For this review, take the finished solid that the model builds, in its own axes (mm). A direction names the side the tool comes from. Round coordinates to 2 decimals unless told otherwise and drop trailing zeros. Write each loop counter-clockwise with the first axis right and the second up, starting at its lowest first coordinate (ties: lowest second). Pieces come first, ordered by that corner, then holes. Notation, with made-up numbers: (43, 20.25) -> (51, 20.25) arc R22 cw to (51, 58.25) -> close; hole circle Ø7 at (33.25, 29). An arc over 180 degrees is marked (long way). Answer in a Markdown table with one row per item.
from build123d import *

# Parameters (mm, degrees)
SKETCH2_W               = 127
SKETCH2_H               = 63.5
BOSS_EXTRUDE1_DEPTH     = 63.5
SHELL1_T                = -2.54
CUT_EXTRUDE1_DEPTH      = 25.4
CUT_EXTRUDE1_DEPTH_BACK = 25.4
CUT_EXTRUDE2_DEPTH      = 52.07
CUT_EXTRUDE2_DEPTH_BACK = 1.27
SKETCH5_R               = 0.3175
FILLET1_R               = 1.27


with BuildPart() as part:
    # Sketch2 → Boss-Extrude1 (new body)
    with BuildSketch(Plane(origin=(0, 0, 0), x_dir=(1, 0, 0), z_dir=(0, 1, 0))):
        Rectangle(SKETCH2_W, SKETCH2_H)
    extrude(amount=BOSS_EXTRUDE1_DEPTH)

    # Shell1
    shell1_openings = [part.faces().sort_by_distance(p)[0] for p in [
        (0, 63.5, 0),
    ]]
    offset(amount=SHELL1_T, openings=shell1_openings, kind=Kind.INTERSECTION)

    # Sketch4 → Cut-Extrude1 (cut, two sides: drawn at the far end of the back side and taken through both)
    with BuildSketch(Plane.XY.offset(-CUT_EXTRUDE1_DEPTH_BACK)):
        with BuildLine():
            Line((-60.96, 63.5), (-63.5, 63.5))
            Line((-63.5, 63.5), (-63.5, 60.96))
            ThreePointArc((-63.5, 60.96), (-61.703948776, 61.703948776), (-60.96, 63.5))
        make_face()
    extrude(amount=CUT_EXTRUDE1_DEPTH + CUT_EXTRUDE1_DEPTH_BACK, mode=Mode.SUBTRACT)

    # Sketch5 → Cut-Extrude2 (cut, two sides: drawn at the far end of the back side and taken through both)
    with BuildSketch(Plane.XY.offset(-25.4).offset(-CUT_EXTRUDE2_DEPTH_BACK)):
        with Locations((-62.5475, 62.5475)):
            Circle(SKETCH5_R)
    extrude(amount=CUT_EXTRUDE2_DEPTH + CUT_EXTRUDE2_DEPTH_BACK, mode=Mode.SUBTRACT)

    # Fillet1
    fillet1_edges = [part.edges().sort_by_distance(p)[0] for p in [
        (-63.5, 63.5, -28.575),
        (-63.5, 63.5, 28.575),
    ]]
    fillet(fillet1_edges, radius=FILLET1_R)


solid = part.part
1) Mouldability with a two-part tool opening along X and no side actions: class faces 1 (the flat face through (-60.96, 33, 0)), 2 (the flat face through (-63.5, 31, 0)), 3 (the flat face through (-62, 62, 25.4)), 4 (the flat face through (63.5, 31, 0)) as pulls with the +X half, pulls with the -X half, needs draft (parallel to the pull), parting line crosses it, or undercut.
Solved:
| item | result |
|---|---|
| face 1 | undercut |
| face 2 | pulls with the -X half |
| face 3 | needs draft |
| face 4 | pulls with the +X half |
2) Consider section B-B on x = -40. State the section outline as (y, z) points.
Solved:
| item | result |
|---|---|
| outline | (0, -31.75) -> (63.5, -31.75) -> (63.5, -29.21) -> (2.54, -29.21) -> (2.54, 29.21) -> (63.5, 29.21) -> (63.5, 31.75) -> (0, 31.75) -> close |
3) Clearance check with a flat-ended pin moving along its axis: pin 1 Ø6 at (x, z) = (16, -1) entering from +Y. State where the tip first meets the part, or that it passes through.
Solved:
| item | result |
|---|---|
| pin 1 | y = 2.54 |
4) Consider section A-A on y = 19. State the section outline as (x, z) points, then the cut area to 3 significant figures.
Solved:
| item | result |
|---|---|
| outline | (-63.5, -31.75) -> (63.5, -31.75) -> (63.5, 31.75) -> (-63.5, 31.75) -> close; hole (-60.96, -29.21) -> (60.96, -29.21) -> (60.96, 29.21) -> (-60.96, 29.21) -> close |
| area | 942 mm² |
5) For faces 5 (the flat face through (-1, 31, -31.75)), 6 (the flat face through (60.96, 33, 0)), 7 (the cylindrical face through (-61.724, 61.684, -0.356)), list the 3-axis set-ups (+Z, -Z, +X, -X, +Y, -Y) from which the entire face can be reached by the end or side of a thin tool; tool diameter is ignored.
Solved:
| item | result |
|---|---|
| face 5 | -Z, +X, -X, +Y, -Y |
| face 6 | +Y |
| face 7 | -X, +Y |
6) For line 1 (Z direction, x = -55.5, y = 20.5); line 2 (X direction, y = 26, z = 9.5); line 3 (Y direction, x = -26, z = -5), list the stretches that pass through material, from the lowest coordinate up. Write a range as [from, to].
Solved:
| item | result |
|---|---|
| line 1 | [-31.75, -29.21], [29.21, 31.75] |
| line 2 | [-63.5, -60.96], [60.96, 63.5] |
| line 3 | [0, 2.54] |
7) Consider section C-C on z = -15. State the section outline as (x, y) points, then the cut area to 3 significant figures.
Solved:
| item | result |
|---|---|
| outline | (-63.5, 0) -> (63.5, 0) -> (63.5, 63.5) -> (60.96, 63.5) -> (60.96, 2.54) -> (-60.96, 2.54) -> (-60.96, 63.5) arc R2.54 cw to (-63.5, 60.96) -> close |
| area | 627 mm² |
